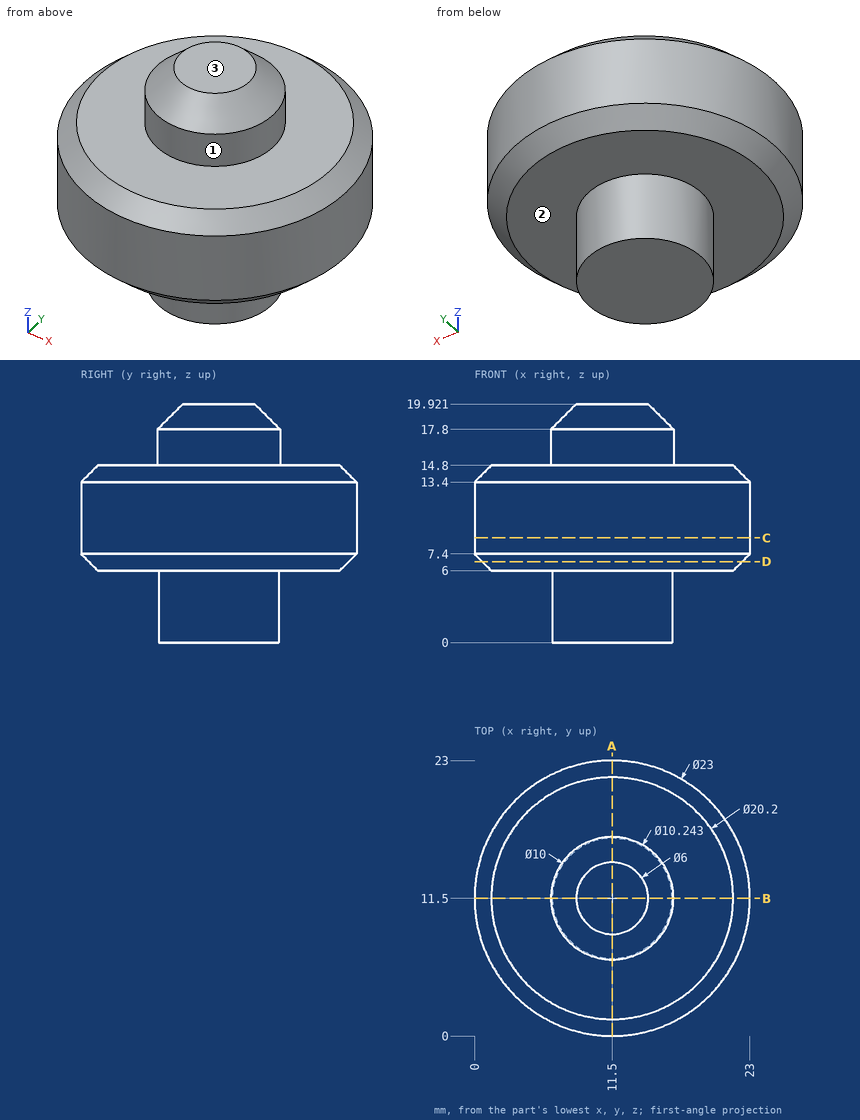
Verification items for this drawing (mm, ordinates from the low corner). A direction names the side the tool comes from. Coordinates: 2 decimals unless noted, no trailing zeros. Order: outer loops, then holes, each group sorted by start corner. A loop starts at its lowest first (then second) coordinate and runs counter-clockwise, first axis right, second up. Notation, with made-up numbers: (52, 37.25) - (70, 37.25) arc R5 cw to (70, 43.25) - close; hole circle Ø2 at (24.5, 19.25). An arc over 180 degrees is marked (long way). Answer in a Markdown table with one row per item. Add a question column.
1. Section check A-A (x = 11.5). Enter the section's corners in (y, z), plus the area to 3 significant figures.
2. Section check D-D (z = 6.75). Enter the section's corners in (x, y).
3. Access from +Z, -Z, +X, -X, +Y, -Y to the whole of each face (thin tool, end or side, straight path). Record for the marked faces 1, 2 and 3.
4. Section check C-C (z = 8.75). Enter the section's corners in (x, y).
5. Gauge pin test, flat ends, axial feed: pin 1 Ø4 at (y, z) = (19.5, 6.5) entering from +X; pin 2 Ø4 at (x, y) = (19.5, 19) entering from -Z; pin 3 Ø6 at (x, z) = (9.5, 3.5) entering from -Y. Record the tip position at first contact, or that the pin passes through.
6. Material ranges on L1, parallel to Z at x = 15, y = 4.25; L2, parallel to Y at x = 16, z = 14.5 (1 decimal); L3, parallel to Y at x = 11.5, z = 15.25, recorded low to high. Write a range as [from, to].
Data:
| question | item | result |
|---|---|---|
| 1 | outline | (0, 7.4) - (1.4, 6) - (6.5, 6) - (6.5, 0) - (16.5, 0) - (16.5, 6) - (21.6, 6) - (23, 7.4) - (23, 13.4) - (21.6, 14.8) - (16.62, 14.8) - (16.62, 17.8) - (14.5, 19.92) - (8.5, 19.92) - (6.38, 17.8) - (6.38, 14.8) - (1.4, 14.8) - (0, 13.4) - close |
| 1 | area | 306 mm² |
| 2 | outline | circle Ø21.7 at (11.5, 11.5) |
| 3 | face 1 | +Z |
| 3 | face 2 | -Z |
| 3 | face 3 | +Z, +X, -X, +Y, -Y |
| 4 | outline | circle Ø23 at (11.5, 11.5) |
| 5 | pin 1 | stops at x = 21.18 |
| 5 | pin 2 | stops at z = 6 |
| 5 | pin 3 | stops at y = 1.05 |
| 6 | L1 | z = [6, 14.8] |
| 6 | L2 | y = [2.1, 20.9] |
| 6 | L3 | y = [6.38, 16.62] |
